from build123d import *

# Parameters (mm, degrees)
SKETCH2_R           = 5
SKETCH2_R_2         = 1.5
BOSS_EXTRUDE1_DEPTH = 2
SKETCH3_R           = 4
SKETCH3_R_2         = 2.5
CUT_EXTRUDE1_DEPTH  = 0.5
CHAMFER1_SIZE       = 0.2
FILLET1_R           = 0.1


with BuildPart() as part:
    # Sketch2 → Boss-Extrude1 (new body, symmetric)
    with BuildSketch(Plane(origin=(0, 0, 0), x_dir=(1, 0, 0), z_dir=(0, 1, 0))):
        Circle(SKETCH2_R)
        Circle(SKETCH2_R_2, mode=Mode.SUBTRACT)
    extrude(amount=BOSS_EXTRUDE1_DEPTH, both=True)

    # Sketch3 → Cut-Extrude1 (cut)
    with BuildSketch(Plane(origin=(0, 2, 0), x_dir=(1, 0, 0), z_dir=(0, 1, 0))):
        Circle(SKETCH3_R)
        Circle(SKETCH3_R_2, mode=Mode.SUBTRACT)
    cut_extrude1 = extrude(amount=-CUT_EXTRUDE1_DEPTH, mode=Mode.SUBTRACT)

    # Mirror1: Cut-Extrude1 across plane
    add(cut_extrude1.mirror(Plane.ZX), mode=Mode.SUBTRACT)

    # Chamfer1
    chamfer1_edges = [part.edges().sort_by_distance(p)[0] for p in [
        (-4, 2, 0),
        (-2.5, 2, 0),
        (-2.5, -2, 0),
        (-4, -2, 0),
    ]]
    chamfer(chamfer1_edges, length=CHAMFER1_SIZE)

    # Fillet1
    fillet1_edges = [part.edges().sort_by_distance(p)[0] for p in [
        (-5, -2, 0),
        (-5, 2, 0),
    ]]
    fillet(fillet1_edges, radius=FILLET1_R)


solid = part.part
Check sheet for the modelled part. Datum: model origin and axes. Units: mm. A direction names the side the tool comes from. Round coordinates to 2 decimals unless told otherwise and drop trailing zeros. Loops run counter-clockwise (first coordinate to the right, second up) from the corner with the lowest first, then second, coordinate; pieces in that order, holes last.
1. Scan lines: probe 1 along Z at (x, y) = (0, -1.55); probe 2 along X at (y, z) = (0.1, 0). Record each from-to range of solid material in increasing order.
2. Mould release check, pull along X, two halves, no side actions. Record for faces 4 (the flat face through (2, 1.5, -2)), 5 (the flat face through (4, -2, -2)), 6 (the cylindrical face through (-1.08, 0.03, 4.88)): released by +X, released by -X, zero draft, split by the parting line, or undercut.
3. Sectioned sample at A-A on y = 0.15. Record the boundary of the cut face in (x, z).
4. Gauge pin test, flat ends, axial feed: pin 1 Ø4 at (x, z) = (0, 0) entering from +Y; pin 2 Ø1.5 at (y, z) = (-0.5, -1.5) entering from +X. Record the tip position at first contact, or that the pin passes through.
5. Set-up check for faces 1 (the cylindrical face through (-0.54, 1.65, 2.44)), 2 (the cylindrical face through (-1.5, -0.03, -0.07)), 3 (the flat face through (2, -1.5, -2)): record each of +Z, -Z, +X, -X, +Y, -Y from which the full face is reachable in a straight line by a thin tool's end or side.
Recorded:
1. probe 1: z = -5 to -4, -2.5 to -1.5, 1.5 to 2.5, 4 to 5
1. probe 2: x = -5 to -1.5, 1.5 to 5
2. face 4: undercut
2. face 5: zero draft
2. face 6: split by the parting line
3. outline: circle Ø10 at (0, 0); hole circle Ø3 at (0, 0)
4. pin 1: stops at y = 2
4. pin 2: stops at x = 4.94
5. face 1: +Y
5. face 2: +Y, -Y
5. face 3: -Y
